Model file for the job. Use its own axes, mm. Face numbers are marked on the shaded views. A direction names the side the tool comes from. Coordinates: 2 decimals unless noted, no trailing zeros. Order: outer loops, then holes, each group sorted by start corner. A loop starts at its lowest first (then second) coordinate and runs counter-clockwise, first axis right, second up. Notation, with made-up numbers: (-28, 22.25) - (-20, 22.25) arc R19 cw to (-20, 48.25) - close; hole circle Ø9 at (53, -16). An arc over 180 degrees is marked (long way). Put each result on its own line as item: value. Start each with the question number.
```python
from build123d import *

# Parameters (mm, degrees)
BOSS_EXTRUDE1_DEPTH = 5
BOSS_EXTRUDE2_DEPTH = 50
CUT_EXTRUDE2_REACH  = 258.619
CIRPATTERN1_COUNT   = 12


with BuildPart() as part:
    # Sketch1 → Boss-Extrude1 (new body)
    with BuildSketch(Plane(origin=(0, 0, 0), x_dir=(1, 0, 0), z_dir=(0, 1, 0))):
        Polygon((-51.086301889, 175.201860999), (-20.896575472, 74.123378061), (-53.744440679, 55.158654242), (-126.186111471, 131.84296572), (-129.77241336, 129.77241336), (-131.84296572, 126.186111471), (-55.158654242, 53.744440679), (-74.123378061, 20.896575472), (-175.201860999, 51.086301889), (-177.27241336, 47.5), (-177.27241336, 43.358895278), (-74.641016151, 18.96472382), (-74.641016151, -18.96472382), (-177.27241336, -43.358895278), (-177.27241336, -47.5), (-175.201860999, -51.086301889), (-74.123378061, -20.896575472), (-55.158654242, -53.744440679), (-131.84296572, -126.186111471), (-129.77241336, -129.77241336), (-126.186111471, -131.84296572), (-53.744440679, -55.158654242), (-20.896575472, -74.123378061), (-51.086301889, -175.201860999), (-47.5, -177.27241336), (-43.358895278, -177.27241336), (-18.96472382, -74.641016151), (18.96472382, -74.641016151), (43.358895278, -177.27241336), (47.5, -177.27241336), (51.086301889, -175.201860999), (20.896575472, -74.123378061), (53.744440679, -55.158654242), (126.186111471, -131.84296572), (129.77241336, -129.77241336), (131.84296572, -126.186111471), (55.158654242, -53.744440679), (74.123378061, -20.896575472), (175.201860999, -51.086301889), (177.27241336, -47.5), (177.27241336, -43.358895278), (74.641016151, -18.96472382), (74.641016151, 18.96472382), (177.27241336, 43.358895278), (177.27241336, 47.5), (175.201860999, 51.086301889), (74.123378061, 20.896575472), (55.158654242, 53.744440679), (131.84296572, 126.186111471), (129.77241336, 129.77241336), (126.186111471, 131.84296572), (53.744440679, 55.158654242), (20.896575472, 74.123378061), (51.086301889, 175.201860999), (47.5, 177.27241336), (43.358895278, 177.27241336), (18.96472382, 74.641016151), (-18.96472382, 74.641016151), (-43.358895278, 177.27241336), (-47.5, 177.27241336), align=None)
    extrude(amount=BOSS_EXTRUDE1_DEPTH)

    # Sketch2 → Boss-Extrude2 (add)
    with BuildSketch(Plane.XZ):
        Polygon((-20.896575472, 74.123378061), (-48.396575472, 176.754775269), (-47.5, 177.27241336), (-46.46472382, 177.27241336), (-18.96472382, 74.641016151), (18.96472382, 74.641016151), (46.46472382, 177.27241336), (47.5, 177.27241336), (48.396575472, 176.754775269), (20.896575472, 74.123378061), (53.744440679, 55.158654242), (128.875837887, 130.29005145), (129.77241336, 129.77241336), (130.29005145, 128.875837887), (55.158654242, 53.744440679), (74.123378061, 20.896575472), (176.754775269, 48.396575472), (177.27241336, 47.5), (177.27241336, 46.46472382), (74.641016151, 18.96472382), (74.641016151, -18.96472382), (177.27241336, -46.46472382), (177.27241336, -47.5), (176.754775269, -48.396575472), (74.123378061, -20.896575472), (55.158654242, -53.744440679), (130.29005145, -128.875837887), (129.77241336, -129.77241336), (128.875837887, -130.29005145), (53.744440679, -55.158654242), (20.896575472, -74.123378061), (48.396575472, -176.754775269), (47.5, -177.27241336), (46.46472382, -177.27241336), (18.96472382, -74.641016151), (-18.96472382, -74.641016151), (-46.46472382, -177.27241336), (-47.5, -177.27241336), (-48.396575472, -176.754775269), (-20.896575472, -74.123378061), (-53.744440679, -55.158654242), (-128.875837887, -130.29005145), (-129.77241336, -129.77241336), (-130.29005145, -128.875837887), (-55.158654242, -53.744440679), (-74.123378061, -20.896575472), (-176.754775269, -48.396575472), (-177.27241336, -47.5), (-177.27241336, -46.46472382), (-74.641016151, -18.96472382), (-74.641016151, 18.96472382), (-177.27241336, 46.46472382), (-177.27241336, 47.5), (-176.754775269, 48.396575472), (-74.123378061, 20.896575472), (-55.158654242, 53.744440679), (-130.29005145, 128.875837887), (-129.77241336, 129.77241336), (-128.875837887, 130.29005145), (-53.744440679, 55.158654242), align=None)
        Polygon((-19.330127019, 72.141016151), (-52.810889132, 52.810889132), (-72.141016151, 19.330127019), (-72.141016151, -19.330127019), (-52.810889132, -52.810889132), (-19.330127019, -72.141016151), (19.330127019, -72.141016151), (52.810889132, -52.810889132), (72.141016151, -19.330127019), (72.141016151, 19.330127019), (52.810889132, 52.810889132), (19.330127019, 72.141016151), align=None, mode=Mode.SUBTRACT)
    extrude(amount=BOSS_EXTRUDE2_DEPTH)

    # Sketch4 → Cut-Extrude2 (cut, up to next)
    with BuildSketch(Plane(origin=(0.7071067811855712, 0, 0.7071067811855722), x_dir=(0.7071067811865479, 0, -0.7071067811865471), z_dir=(0.7071067811865471, 0, 0.7071067811865479)), mode=Mode.PRIVATE) as cut_extrude2_sk1:
        Polygon((-77.006116911, -50), (-183.136497491, 0), (-183.257957802, 0), (-183.257957802, -50), align=None)
    cut_extrude2_tool1 = extrude(cut_extrude2_sk1.sketch, amount=-CUT_EXTRUDE2_REACH, mode=Mode.PRIVATE) & part.part
    # Sketch4 → Cut-Extrude2 (cut, up to next)
    with BuildSketch(Plane(origin=(0.7071067811855712, 0, 0.7071067811855722), x_dir=(0.7071067811865479, 0, -0.7071067811865471), z_dir=(0.7071067811865471, 0, 0.7071067811865479)), mode=Mode.PRIVATE) as cut_extrude2_sk2:
        Polygon((-183.136497491, 0), (-185.006116911, 0.880812549), (-185.006116911, -50), (-183.257957802, -50), (-183.257957802, 0), align=None)
    cut_extrude2_tool2 = extrude(cut_extrude2_sk2.sketch, amount=-CUT_EXTRUDE2_REACH, mode=Mode.PRIVATE) & part.part
    cut_extrude2_1 = cut_extrude2_tool1.solids().sort_by_distance((-103.832006, -33.314303, 105.24622))[0]
    add(cut_extrude2_1, mode=Mode.SUBTRACT)
    cut_extrude2_2 = cut_extrude2_tool2.solids().sort_by_distance((-129.495561, -24.763955, 130.909775))[0]
    add(cut_extrude2_2, mode=Mode.SUBTRACT)
    cut_extrude2 = cut_extrude2_1 + cut_extrude2_2  # Cut-Extrude2 as one shape, for the pattern or mirror that repeats it

    # CirPattern1: Cut-Extrude2 ×12 about axis
    cirpattern1_axis = Axis((0, 0, 0), (0, 1, 0))
    for i in range(1, CIRPATTERN1_COUNT):
        add(cut_extrude2.rotate(cirpattern1_axis, i * 360 / CIRPATTERN1_COUNT), mode=Mode.SUBTRACT)


solid = part.part
```
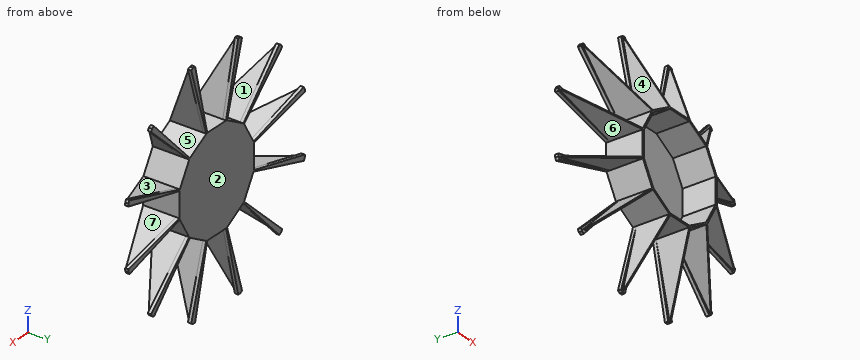
Item 1: Flat gauge pins, fed straight in: pin 1 Ø15 at (x, z) = (-148.5, 43) entering from -Y; pin 2 Ø10 at (x, y) = (-108, -26.5) entering from +Z; pin 3 Ø5 at (x, y) = (78, -23.5) entering from +Z. Where does each tip first touch, or does it go through?
Item 2: Slice it at D-D, the plane z = -154. Give the cut face in (x, y).
Item 3: Pull direction Z, two halves, no side cores. Call the marked faces 1, 2 and 3: pulls with the +Z half, pulls with the -Z half, needs draft (parallel to the pull), parting line crosses it, or undercut.
Item 4: Slice it at A-A, the plane x = -12.5. Give the cut face in (y, z).
Item 5: 3-axis set-ups, long thin cutter, end or side, ignore diameter. For the marked faces 4, 5, 6 and 7: which of +Z, -Z, +X, -X, +Y, -Y reach the whole face in a straight line?
Item 6: Wall check: line 1 along Z through (x, y) = (-7.5, -40); line 2 along X through (y, z) = (-15, 82.5); line 3 along Z through (x, y) = (-62.5, -33). Give the ranges that are in metal, low to high.
Item 7: Slice it at C-C, the plane x = 148. Give the cut face in (y, z), plus the area to 3 significant figures.
Item 8: Slice it at B-B, the plane z = 101. Give the number of separate pieces and of enclosed holes in the cut face, plus the area to 3 significant figures.
Here are the results:
1. pin 1: stops at y = -16.85
1. pin 2: stops at z = 31.31
1. pin 3: stops at z = 81.91
2. outline: (-44.75, 0) - (-42.3, 0) - (-42.3, -11.04) - (-40.23, -11.29) - (-40.23, 0) - (-37.83, 0) - (-37.83, 5) - (-44.75, 5) - close; (37.83, 0) - (40.23, 0) - (40.23, -11.29) - (42.3, -11.04) - (42.3, 0) - (44.75, 0) - (44.75, 5) - (37.83, 5) - close
3. face 1: pulls with the +Z half
3. face 2: needs draft
3. face 3: undercut
4. outline: (-50, -74.64) - (5, -74.64) - (5, 74.64) - (-50, 74.64) - (-50, 72.14) - (0, 72.14) - (0, -72.14) - (-50, -72.14) - close
5. face 4: -Y
5. face 5: +Y, -Y
5. face 6: -X, -Y
5. face 7: +X, -Y
6. line 1: z = -74.64 to -72.14, 72.14 to 74.64
6. line 2: x = -83.91 to -81.09, -23.14 to -21.07, 21.07 to 23.14, 81.09 to 83.91
6. line 3: z = -63.91 to -61.09, -41.03 to -36.03, 36.03 to 41.03, 61.09 to 63.91
7. outline: (-14.22, -38.62) - (-13.97, -40.69) - (0, -40.69) - (0, -42.96) - (5, -42.96) - (5, -36.4) - (0, -36.4) - (0, -38.62) - close; (-14.22, 38.62) - (0, 38.62) - (0, 36.4) - (5, 36.4) - (5, 42.96) - (0, 42.96) - (0, 40.69) - (-13.97, 40.69) - close
7. area: 124 mm^2
8. separate pieces: 4
8. enclosed holes: 0
8. area: 379 mm^2
